Source: CAD feature listing. Evaluate the final solid. Frame: model axes, mm. A direction names the side the tool comes from. Coordinates: 2 decimals unless noted, no trailing zeros. Write each loop counter-clockwise with the first axis right and the second up, starting at its lowest first coordinate (ties: lowest second). Pieces come first, ordered by that corner, then holes. Notation, with made-up numbers: M 16.5,-18 L 27.5,-18 A26 ccw 27.5,16 Z; hole C -4.75,54 d1. An arc over 180 degrees is marked long. Answer as CSV lines item,"result". Start each with the question number.
1. Line query: probe 1 along Y at (x, z) = (0.25, 21.5); probe 2 along Y at (x, z) = (6.85, 134); probe 3 along Y at (x, z) = (-6.75, 122.5). Output: solid intervals per line, ascending. Write a range as [from, to].
2. Mould query, pull axis X, two halves, no side actions, for faces 4 (the face through (-4, -20, 79)), 5 (the face through (6.958, 1.201, 137.815)), 6 (the face through (-7.05, 34, 79)). Classes: pulls with the +X half, pulls with the -X half, needs draft (parallel to the pull), parting line crosses it, or undercut.
3. Section D-D on y = -17.5. Return the cut outline in (x, z), plus the area to 3 significant figures.
4. Section C-C on y = 0. Return the cut outline in (x, z), plus the area to 3 significant figures.
5. Reachability of faces 1 (the face through (8, -15.85, 79)), 2 (the face through (3, -12.95, 79)), 3 (the face through (-8, 4.15, 122)) from +Z, -Z, +X, -X, +Y, -Y: full face, straight path, thin tool, end or side. Return the list, or none.
6. Section A-A on x = -1.5. Return the cut outline in (y, z), plus the area to 3 significant figures.
7. Section B-B on y = -31.5. Return the cut outline in (x, z).
8. Contact query for flat-ended pins moving along their axis: pin 1 Ø7 at (y, z) = (0, 134) entering from -X; pin 2 Ø2.5 at (y, z) = (2, 123.5) entering from -X; pin 3 Ø2 at (x, z) = (1.5, 38.5) entering from +Y. Output: stop coordinate, or through.
```python
from build123d import *

# Parameters (mm, degrees)
EXTRUDE_1_DEPTH           = 160
HOLE_WIZARD_8_0_8_1_D     = 8
HOLE_WIZARD_8_0_8_2_D     = 8
HOLE_WIZARD_8_0_8_2_DEPTH = 8
HOLE_WIZARD_8_0_8_2_TIP   = 2.403442476
HOLE_WIZARD_12_0_12_2_D   = 12


with BuildPart() as part:
    # Sketch1 → 凸台-拉伸1 (new body)
    with BuildSketch(Plane.XY):
        with BuildLine():
            Line((-9, 40), (-4.15, 40))
            Line((-4.15, 40), (-4.15, 37))
            Line((-4.15, 37), (-7.05, 37))
            Line((-7.05, 37), (-7.05, 30))
            Line((-7.05, 30), (7.05, 30))
            Line((7.05, 30), (7.05, 37))
            Line((7.05, 37), (4.15, 37))
            Line((4.15, 37), (4.15, 40))
            Line((4.15, 40), (9, 40))
            ThreePointArc((9, 40), (9.707106781, 39.707106781), (10, 39))
            Line((10, 39), (10, 24.15))
            Line((10, 24.15), (6, 24.15))
            Line((6, 24.15), (6, 27.05))
            Line((6, 27.05), (0, 27.05))
            Line((0, 27.05), (0, 24.15))
            Line((0, 24.15), (-4, 24.15))
            Line((-4, 24.15), (-4, 15.85))
            Line((-4, 15.85), (0, 15.85))
            Line((0, 15.85), (0, 12.95))
            Line((0, 12.95), (6, 12.95))
            Line((6, 12.95), (6, 15.85))
            Line((6, 15.85), (10, 15.85))
            Line((10, 15.85), (10, -15.85))
            Line((10, -15.85), (6, -15.85))
            Line((6, -15.85), (6, -12.95))
            Line((6, -12.95), (0, -12.95))
            Line((0, -12.95), (0, -15.85))
            Line((0, -15.85), (-4, -15.85))
            Line((-4, -15.85), (-4, -24.15))
            Line((-4, -24.15), (0, -24.15))
            Line((0, -24.15), (0, -27.05))
            Line((0, -27.05), (6, -27.05))
            Line((6, -27.05), (6, -24.15))
            Line((6, -24.15), (10, -24.15))
            Line((10, -24.15), (10, -39))
            ThreePointArc((10, -39), (9.707106781, -39.707106781), (9, -40))
            Line((9, -40), (4.15, -40))
            Line((4.15, -40), (4.15, -37))
            Line((4.15, -37), (7.05, -37))
            Line((7.05, -37), (7.05, -30))
            Line((7.05, -30), (-7.05, -30))
            Line((-7.05, -30), (-7.05, -37))
            Line((-7.05, -37), (-4.15, -37))
            Line((-4.15, -37), (-4.15, -40))
            Line((-4.15, -40), (-9, -40))
            ThreePointArc((-9, -40), (-9.707106781, -39.707106781), (-10, -39))
            Line((-10, -39), (-10, -4.15))
            Line((-10, -4.15), (-6, -4.15))
            Line((-6, -4.15), (-6, -7.05))
            Line((-6, -7.05), (0, -7.05))
            Line((0, -7.05), (0, -4.15))
            Line((0, -4.15), (4, -4.15))
            Line((4, -4.15), (4, 4.15))
            Line((4, 4.15), (0, 4.15))
            Line((0, 4.15), (0, 7.05))
            Line((0, 7.05), (-6, 7.05))
            Line((-6, 7.05), (-6, 4.15))
            Line((-6, 4.15), (-10, 4.15))
            Line((-10, 4.15), (-10, 39))
            ThreePointArc((-10, 39), (-9.707106781, 39.707106781), (-9, 40))
        make_face()
    extrude(amount=EXTRUDE_1_DEPTH)

    # Ø8.0 (8) 直径孔1 (through all)
    with Locations(Plane(origin=(10, 0, 0), x_dir=(0, 0, -1), z_dir=(1, 0, 0))):
        with Locations((-134, 0)):
            Hole(HOLE_WIZARD_8_0_8_1_D / 2)

    # Ø8.0 (8) 直径孔2
    with Locations(Plane(origin=(10, 0, 0), x_dir=(0, 0, -1), z_dir=(1, 0, 0))):
        with Locations((-26, 0)):
            Hole(HOLE_WIZARD_8_0_8_2_D / 2, depth=HOLE_WIZARD_8_0_8_2_DEPTH)
            with Locations((0, 0, -(HOLE_WIZARD_8_0_8_2_DEPTH + HOLE_WIZARD_8_0_8_2_TIP / 2))):  # 118° drill point
                Cone(0, HOLE_WIZARD_8_0_8_2_D / 2, HOLE_WIZARD_8_0_8_2_TIP, mode=Mode.SUBTRACT)

    # Ø12.0 (12) 直径孔2 (through all)
    with Locations(Plane(origin=(10, 0, 0), x_dir=(0, 0, -1), z_dir=(1, 0, 0))):
        with Locations((-80, 0)):
            Hole(HOLE_WIZARD_12_0_12_2_D / 2)


solid = part.part
```
Values:
1,probe 1,"[-30, -27.05], [-12.95, -4.15], [4.15, 12.95], [27.05, 30]"
1,probe 2,"[-40, -37], [-30, -24.15], [-15.85, -4], [4, 15.85], [24.15, 30], [37, 40]"
1,probe 3,"[-40, -37], [-30, -4.15], [4.15, 30], [37, 40]"
2,face 4,"pulls with the +X half"
2,face 5,"needs draft"
2,face 6,"undercut"
3,outline,"M -10,0 L -4,0 L -4,160 L -10,160 Z"
3,area,"960 mm²"
4,outline,"M 4,0 L 10,0 L 10,22 L 4,22 Z; M 4,30 L 10,30 L 10,74 L 4,74 Z; M 4,86 L 10,86 L 10,130 L 4,130 Z; M 4,138 L 10,138 L 10,160 L 4,160 Z"
4,area,"792 mm²"
5,face 1,"+Z, -Z, +X"
5,face 2,"+Z, -Z"
5,face 3,"+Z, -Z, -X"
6,outline,"M -30,0 L -24.15,0 L -24.15,160 L -30,160 Z; M -15.85,0 L -7.05,0 L -7.05,160 L -15.85,160 Z; M 7.05,0 L 15.85,0 L 15.85,160 L 7.05,160 Z; M 24.15,0 L 30,0 L 30,160 L 24.15,160 Z"
6,area,"4,690 mm²"
7,outline,"M -10,0 L -7.05,0 L -7.05,160 L -10,160 Z; M 7.05,0 L 10,0 L 10,160 L 7.05,160 Z"
8,pin 1,"through"
8,pin 2,"x = 4"
8,pin 3,"y = 30"
